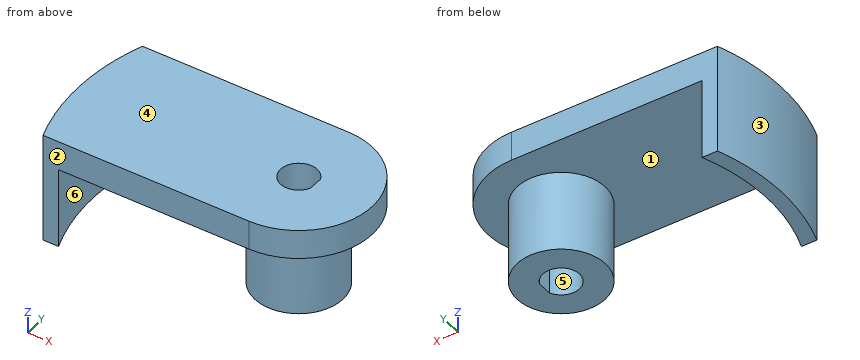
```python
from build123d import *

# Parameters (mm, degrees)
PAD001_DEPTH    = 15
SKETCH004_R     = 28
SKETCH004_R_2   = 6
POCKET001_DEPTH = 11
POCKET002_DEPTH = 15.001


with BuildPart() as part:
    # Sketch003 → Pad001 (new body)
    with BuildSketch(Plane.XY):
        with BuildLine():
            ThreePointArc((0, -10), (10, 0), (0, 10))
            Line((0, 10), (-28.284271, 10))
            ThreePointArc((-28.284271, 10), (-30, 0), (-28.284271, -10))
            Line((0, -10), (-28.284271, -10))
        make_face()
    extrude(amount=PAD001_DEPTH)

    # Sketch004 (on Face5 of Pad001) → Pocket001 (cut)
    with BuildSketch(Plane(origin=(0, 0, 0), x_dir=(1, 0, 0), z_dir=(0, 0, -1))):
        Circle(SKETCH004_R)
        Circle(SKETCH004_R_2, mode=Mode.SUBTRACT)
    extrude(amount=-POCKET001_DEPTH, mode=Mode.SUBTRACT)

    # Sketch005 (on Face10 of Pocket001) → Pocket002 (cut, through all)
    with BuildSketch(Plane(origin=(0, 0, 0), x_dir=(1, 0, 0), z_dir=(0, 0, -1))):
        with BuildLine():
            ThreePointArc((2.291288, 1), (-2.5, 0), (2.291288, -1))
            Line((2.291288, -1), (2.291288, 1))
        make_face()
    extrude(amount=-POCKET002_DEPTH, mode=Mode.SUBTRACT)


solid = part.part
```
Input: part model. Units: mm. Frame: model coordinates. Face numbers are marked on the shaded views. A direction names the side the tool comes from. Round coordinates to 2 decimals unless told otherwise and drop trailing zeros. Order: outer loops, then holes, each group sorted by start corner. A loop starts at its lowest first (then second) coordinate and runs counter-clockwise, first axis right, second up. Notation, with made-up numbers: (-38.5, -22) - (-16.5, -22) arc R33 cw to (-16.5, 17) - close; hole circle Ø3 at (0, -19). An arc over 180 degrees is marked (long way). Answer in a Markdown table with one row per item.
Item 1: Section query C-C (x = -5). Return the cut outline in (y, z), then the cut area to 3 significant figures.
Model answer:
| item | result |
|---|---|
| outline | (-10, 11) - (-3.32, 11) - (-3.32, 0) - (3.32, 0) - (3.32, 11) - (10, 11) - (10, 15) - (-10, 15) - close |
| area | 153 mm² |
Item 2: Mould query, pull axis Y, two halves, no side actions, for the marked faces 3, 4, 5 and 6. Classes: released by +Y, released by -Y, zero draft, split by the parting line, or undercut.
Model answer:
| item | result |
|---|---|
| face 3 | split by the parting line |
| face 4 | zero draft |
| face 5 | undercut |
| face 6 | undercut |
Item 3: Pin query (flat end, axial travel): pin 1 (3 mm diameter, centred on x = 5, z = 7.5, fed in from -Y); pin 2 (5 mm diameter, centred on x = -14.5, y = 3.5, fed in from -Z); pin 3 (2 mm diameter, centred on y = 0, z = 4, fed in from -X). Return the tip coordinate at first contact, or that it passes through.
Model answer:
| item | result |
|---|---|
| pin 1 | stops at y = -4.87 |
| pin 2 | stops at z = 11 |
| pin 3 | stops at x = -30 |
Item 4: Line query: line 1 (X direction, y = 0, z = 7.5); line 2 (X direction, y = -2, z = 2.75); line 3 (Y direction, x = 0, z = 5.5). Output: solid intervals per line, ascending.
Model answer:
| item | result |
|---|---|
| line 1 | x = -30 to -28, -6 to -2.5, 2.29 to 6 |
| line 2 | x = -29.93 to -27.93, -5.66 to -1.5, 1.5 to 5.66 |
| line 3 | y = -6 to -2.5, 2.5 to 6 |
Item 5: Section query A-A (z = 5.75). Return the cut outline in (x, y).
Model answer:
| item | result |
|---|---|
| outline | (-28.28, -10) - (-26.15, -10) arc R28 cw to (-26.15, 10) - (-28.28, 10) arc R30 ccw to start; circle Ø12 at (0, 0); hole (2.29, -1) - (2.29, 1) arc R2.5 ccw (long way) to start |
Item 6: Reachability of the marked faces 1 and 2 from +Z, -Z, +X, -X, +Y, -Y: full face, straight path, thin tool, end or side. Return the list, or none.
Model answer:
| item | result |
|---|---|
| face 1 | -Z |
| face 2 | +Z, -Z, +X, -X, -Y |
Item 7: Section query D-D (y = -7.25). Return the cut outline in (x, z), then the cut area to 3 significant figures.
Model answer:
| item | result |
|---|---|
| outline | (-29.11, 0) - (-27.05, 0) - (-27.05, 11) - (6.89, 11) - (6.89, 15) - (-29.11, 15) - close |
| area | 167 mm² |
Item 8: Section query B-B (y = 0). Return the cut outline in (x, z), then the cut area to 3 significant figures.
Model answer:
| item | result |
|---|---|
| outline | (-30, 0) - (-28, 0) - (-28, 11) - (-6, 11) - (-6, 0) - (-2.5, 0) - (-2.5, 15) - (-30, 15) - close; (2.29, 0) - (6, 0) - (6, 11) - (10, 11) - (10, 15) - (2.29, 15) - close |
| area | 242 mm² |
